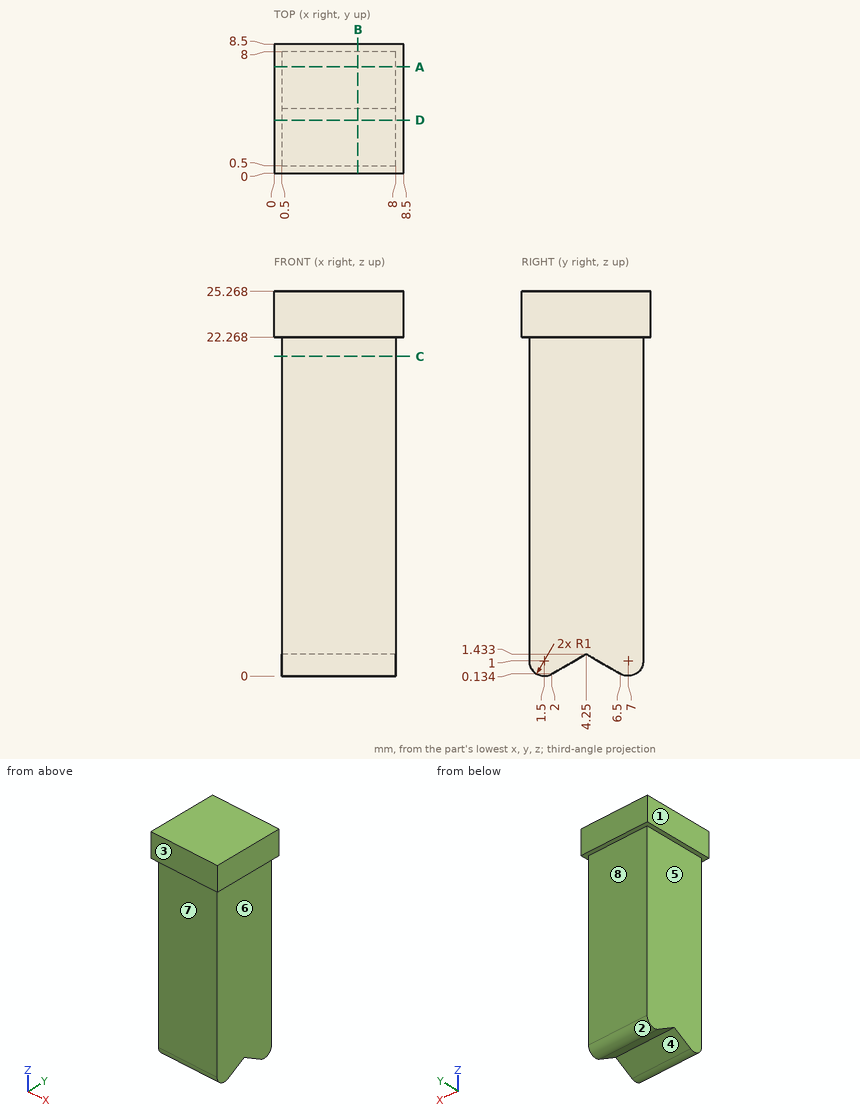
For this review, use the dimensioned drawing (mm, ordinates from the lowest corner) and the shaded views. A direction names the side the tool comes from. Coordinates: 2 decimals unless noted, no trailing zeros. Write each loop counter-clockwise with the first axis right and the second up, starting at its lowest first coordinate (ties: lowest second). Pieces come first, ordered by that corner, then holes. Notation, with made-up numbers: (36.5, -7) -> (87.5, -7) arc R36 ccw to (87.5, 27) -> close; hole circle Ø11 at (81.5, 24). An arc over 180 degrees is marked (long way). Write each question's results on one line, items separated by ' | '. Start each with the question number.
(1) Take a section at A-A on y = 7. Write out the cut boundary in (x, z).
(2) Take a section at B-B on x = 5.5. Write out the cut boundary in (y, z).
(3) For line 1 along Z through (x, y) = (1.75, 8.25); line 2 along Z through (x, y) = (6.75, 7.5); line 3 along X through (y, z) = (2.75, 8.75), list the stretches that pass through material, from the lowest coordinate up. Write a range as from..to.
(4) Take a section at C-C on z = 21. Write out the cut boundary in (x, y).
(5) Take a section at D-D on y = 3.5. Write out the cut boundary in (x, z), and give its area (3 significant figures).
(6) Clearance check with flat-ended pins moving along their axes: P1, Ø4, axis at x = 7, z = 13.5, coming from the +Y side; P2, Ø2, axis at x = 2.5, z = 10, coming from the -Y side; P3, Ø4, axis at y = 4.5, z = 15, coming from the +X side. State where each tip first meets the part, or that it passes through.
(7) The part is to be moulded in two halves that separate along Y. For the marked faces 1, 2 and 3, say which applies: pulls with the +Y half, pulls with the -Y half, needs draft (parallel to the pull), parting line crosses it, or undercut.
(8) Tool access review of the marked faces 4, 5, 6, 7 and 8: name each direction out of +Z, -Z, +X, -X, +Y, -Y from which nothing blocks a thin tool from reaching the whole face with its end or side.
Results found:
1) outline: (0, 22.27) -> (0.5, 22.27) -> (0.5, 0) -> (8, 0) -> (8, 22.27) -> (8.5, 22.27) -> (8.5, 25.27) -> (0, 25.27) -> close
2) outline: (0, 22.27) -> (0.5, 22.27) -> (0.5, 1) arc R1 ccw to (2, 0.13) -> (4.25, 1.43) -> (6.5, 0.13) arc R1 ccw to (8, 1) -> (8, 22.27) -> (8.5, 22.27) -> (8.5, 25.27) -> (0, 25.27) -> close
3) line 1: z = 22.27..25.27 | line 2: z = 0.13..25.27 | line 3: x = 0.5..8
4) outline: (0.5, 0.5) -> (8, 0.5) -> (8, 8) -> (0.5, 8) -> close
5) outline: (0, 22.27) -> (0.5, 22.27) -> (0.5, 1) -> (8, 1) -> (8, 22.27) -> (8.5, 22.27) -> (8.5, 25.27) -> (0, 25.27) -> close | area: 185 mm2
6) P1: stops at y = 8 | P2: stops at y = 0.5 | P3: stops at x = 8
7) face 1: needs draft | face 2: undercut | face 3: pulls with the -Y half
8) face 4: -Z, +X, -X | face 5: -Z, -X, +Y, -Y | face 6: -Z, +X, +Y, -Y | face 7: -Z, +X, -X, -Y | face 8: -Z, +X, -X, +Y
